Geometry check sheet. Reference: drawing and pictorial views, mm from the part's lowest x, y, z. A direction names the side the tool comes from. Give positions to 0.01 mm unless a question says otherwise; leave off trailing zeros. Order: outer loops, then holes, each group sorted by start corner. A loop starts at its lowest first (then second) coordinate and runs counter-clockwise, first axis right, second up.
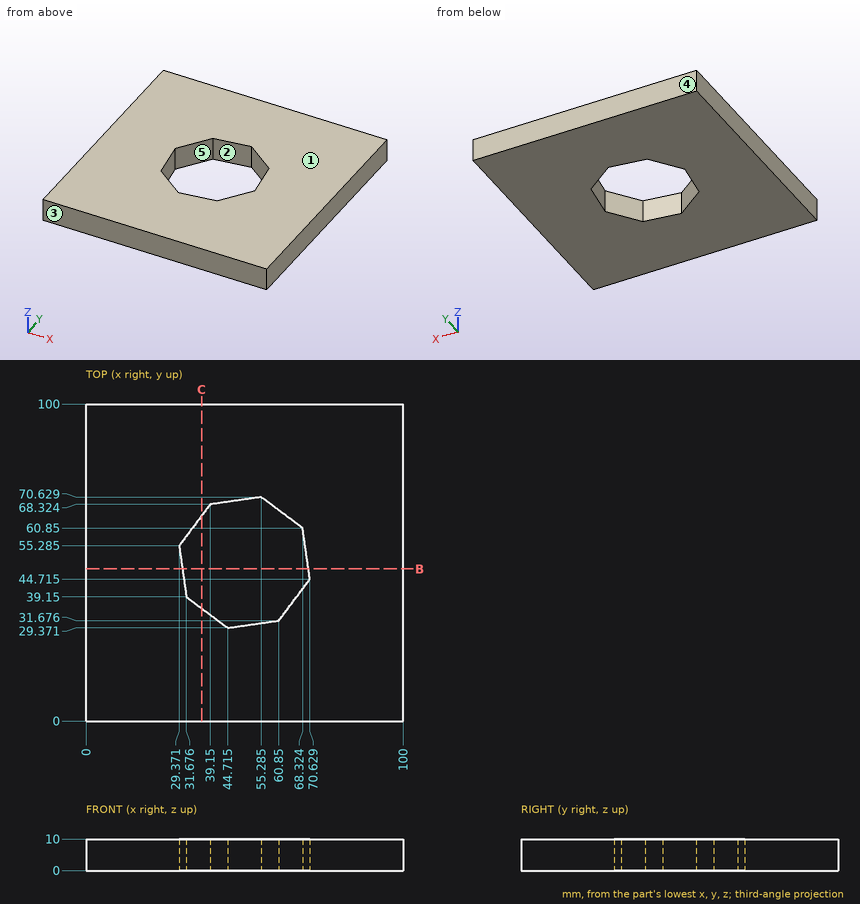
1) Set-up check for the marked faces 4 and 5: record each of +Z, -Z, +X, -X, +Y, -Y from which the full face is reachable in a straight line by a thin tool's end or side.
Recorded:
face 4: +Z, -Z, +X, -X, +Y
face 5: +Z, -Z
2) Depth check by flat-ended pin: pin 1 Ø5 at (x, z) = (61.5, 8.5) entering from -Y. Enter the tip coordinate at first touch or a pass-through.
Recorded:
pin 1: stops at y = 0
3) Section check B-B, the plane y = 48. Record the cut outline in (x, z).
Recorded:
outline: (0, 0) - (30.41, 0) - (30.41, 10) - (0, 10) - close; (70.16, 0) - (100, 0) - (100, 10) - (70.16, 10) - close
4) Section check C-C, the plane x = 36.5. Record the cut outline in (y, z).
Recorded:
outline: (0, 0) - (35.53, 0) - (35.53, 10) - (0, 10) - close; (64.79, 0) - (100, 0) - (100, 10) - (64.79, 10) - close
5) Material ranges on L1, parallel to X at y = 42, z = 5.5 (1 decimal); L2, parallel to Y at x = 49, z = 2.5; L3, parallel to Y at x = 50.5, z = 3.5 (1 decimal), recorded low to high.
Recorded:
L1: x = 0 to 31.3, 68.6 to 100
L2: y = 0 to 29.98, 69.73 to 100
L3: y = 0 to 30.2, 69.9 to 100
6) Draft check along Y on the marked faces 1, 2 and 3. Enter one of: +Y half, -Y half, draft (parallel to the pull), parting line (faces both ways), or undercut.
Recorded:
face 1: draft
face 2: undercut
face 3: -Y half
